Can you work these out from the model? Positions are in its coordinate system, mm. A direction names the side the tool comes from. Coordinates: 2 decimals unless noted, no trailing zeros. Loops run counter-clockwise (first coordinate to the right, second up) from the corner with the lowest first, then second, coordinate; pieces in that order, holes last.
```python
from build123d import *

# Parameters (mm, degrees)
F0_W      = 70
F0_H      = 120
F0_W_2    = 66
F0_H_2    = 116
F1_DEPTH  = 6
F0_W_3    = 76
F0_H_3    = 126
F2_DEPTH  = 3
F3_R      = 5
F4_W      = 11.5
F4_H      = 13.5
F5_DEPTH  = 25
F8_W      = 13.5
F8_H      = 1.5
F9_DEPTH  = 1
F6_W      = 11.5
F6_H      = 1.5
F10_DEPTH = 1
F7_W      = 13.5
F7_H      = 1.5
F11_DEPTH = 1
F13_DEPTH = 25
F14_W     = 1
F14_H     = 1.5
F15_W     = 1
F15_H     = 1.5
F16_DEPTH = 3


with BuildPart() as f1:
    # F0 (on Top) → F1 (new body)
    with BuildSketch(Plane.XY):
        Rectangle(F0_W, F0_H)
        Rectangle(F0_W_2, F0_H_2, mode=Mode.SUBTRACT)
    extrude(amount=F1_DEPTH)

    # F0 (on Top) → F2 (join)
    with BuildSketch(Plane.XY):
        Rectangle(F0_W_3, F0_H_3)
        Rectangle(F0_W, F0_H, mode=Mode.SUBTRACT)
        Rectangle(F0_W_2, F0_H_2)
    extrude(amount=F2_DEPTH)

    # F3
    f3_edges = [f1.edges().sort_by_distance(p)[0] for p in [
        (-38, 63, 1.5),
        (38, 63, 1.5),
    ]]
    fillet(f3_edges, radius=F3_R)

    # F4 (on face) → F5 (cut)
    with BuildSketch(Plane.XY.offset(3)):
        with Locations((27.25, -51.25)):
            Rectangle(F4_W, F4_H)
    extrude(amount=-F5_DEPTH, mode=Mode.SUBTRACT)

    # F8 (on face) → F9 (join)
    with BuildSketch(Plane(origin=(33, 0, 0), x_dir=(0, -1, 0), z_dir=(-1, 0, 0))):
        with Locations((51.25, 1.5)):
            Rectangle(F8_W, F8_H)
    extrude(amount=F9_DEPTH)

    # F6 (on face) → F10 (join)
    with BuildSketch(Plane.XZ.offset(44.5)):
        with Locations((27.25, 1.5)):
            Rectangle(F6_W, F6_H)
    extrude(amount=F10_DEPTH)

    # F7 (on face) → F11 (join)
    with BuildSketch(Plane.YZ.offset(21.5)):
        with Locations((-51.25, 1.5)):
            Rectangle(F7_W, F7_H)
    extrude(amount=F11_DEPTH)

    # F12 (on face) → F13 (cut)
    with BuildSketch(Plane(origin=(0, -58, 0), x_dir=(-1, 0, 0), z_dir=(0, 1, 0))):
        Polygon((-21.5, 2.25), (-21.5, 3), (-21.5, 6), (-33, 6), (-33, 2.25), (-32, 2.25), (-32, 0.75), (-33, 0.75), (-33, 0), (-21.5, 0), (-21.5, 0.75), (-22.5, 0.75), (-22.5, 2.25), align=None)
    extrude(amount=-F13_DEPTH, mode=Mode.SUBTRACT)

    # F14 (on face) + F15 (on face) → F16 (cut)
    with BuildSketch(Plane.XZ.offset(63)):
        with Locations((22, 1.5)):
            Rectangle(F14_W, F14_H)
    with BuildSketch(Plane.XZ.offset(63)):
        with Locations((32.5, 1.5)):
            Rectangle(F15_W, F15_H)
    extrude(amount=-F16_DEPTH, mode=Mode.SUBTRACT)


solid = f1.part
```
Item 1: Suppose I cut it at B-B, the plane x = -21. Please give me the cut outline in (y, z).
Results are:
outline: (-63, 0) - (63, 0) - (63, 3) - (60, 3) - (60, 6) - (58, 6) - (58, 3) - (-58, 3) - (-58, 6) - (-60, 6) - (-60, 3) - (-63, 3) - close
Item 2: On a 3-axis mill with a long thin cutter (end or side, diameter ignored), from which of +Z, -Z, +X, -X, +Y, -Y can I reach the whole of each face in a straight line? I mean faces 4 (the face through (-33, -1, 4)), 5 (the face through (35, -1, 4)), 6 (the face through (0, 60, 4)), 7 (the face through (32.3, -50.6, 2.25)). Say none if no direction works.
Results are:
face 4: +Z
face 5: +Z, +X, +Y, -Y
face 6: +Z, +X, -X, +Y
face 7: +Z, -Y
Item 3: I need wall thicknesses on line 1 along Y through (x, z) = (1, 4.05); line 2 along X through (y, z) = (1, 3.65); line 3 along Z through (x, y) = (5, -38.5). Which ranges of each line are inside material? Lowest first, please.
Results are:
line 1: y = -60 to -58, 58 to 60
line 2: x = -35 to -33, 33 to 35
line 3: z = 0 to 3
Item 4: Suppose I cut it at A-A, the plane z = 4. Please give me the cut outline in (x, y).
Results are:
outline: (-35, -60) - (21.5, -60) - (21.5, -58) - (-33, -58) - (-33, 58) - (33, 58) - (33, -60) - (35, -60) - (35, 60) - (-35, 60) - close
Item 5: I'm going to push flat-ended pins straight in: P1, Ø12, axis at x = 8.5, y = 40.5, coming from the -Z side; P2, Ø1.6, axis at x = 34, z = 4, coming from the -Y side; P3, Ø1.5, axis at y = -24, z = 4.5, coming from the +X side; P4, Ø3, axis at x = -22.5, y = 7, coming from the +Z side. Where does each tip first touch, or does it pass through?
Results are:
P1: stops at z = 0
P2: stops at y = -60
P3: stops at x = 35
P4: stops at z = 3
Item 6: Suppose I cut it at C-C, the plane y = 24. Please give me the cut outline in (x, z), plus the area to 3 significant figures.
Results are:
outline: (-38, 0) - (38, 0) - (38, 3) - (35, 3) - (35, 6) - (33, 6) - (33, 3) - (-33, 3) - (-33, 6) - (-35, 6) - (-35, 3) - (-38, 3) - close
area: 240 mm2
Item 7: We'd pull the mould along X, two halves only. Please class faces 1 (the face through (-7, -60, 4)), 2 (the face through (38, -3, 1)), 3 (the face through (21.5, -55.8, 2.6)): +X half, -X half, draft (parallel to the pull), parting line (faces both ways), or undercut.
Results are:
face 1: draft
face 2: +X half
face 3: undercut
